Could you check a few things on this model? Use its own coordinates, in mm. Face numbers are marked on the shaded views. A direction names the side the tool comes from. Round coordinates to 2 decimals unless told otherwise and drop trailing zeros. Loops run counter-clockwise (first coordinate to the right, second up) from the corner with the lowest first, then second, coordinate; pieces in that order, holes last. Notation, with made-up numbers: (23, 46) -> (79, 46) arc R20 ccw to (79, 61) -> close; hole circle Ø6 at (14.5, -32.5). An arc over 180 degrees is marked (long way). One line per item, written item: value.
from build123d import *

# Parameters (mm, degrees)
BOSS_EXTRUDE1_DEPTH = 300
SKETCH3_W           = 90
SKETCH3_H           = 90
BOSS_EXTRUDE2_DEPTH = 70


with BuildPart() as part:
    # Sketch2 → Boss-Extrude1 (new body)
    with BuildSketch(Plane(origin=(0, 0, 0), x_dir=(1, 0, 0), z_dir=(0, 1, 0))):
        Polygon((0, 0), (0, 75), (45, 75), (110.363656587, 121.756282785), (145.853333333, 72.142949451), (45, 0), align=None)
    boss_extrude1 = extrude(amount=BOSS_EXTRUDE1_DEPTH)

    # Mirror1: Boss-Extrude1 across plane
    add(boss_extrude1.mirror(Plane(origin=(0, 0, 0), x_dir=(0, 0, 1), z_dir=(1, 0, 0))))

    # Sketch3 → Boss-Extrude2 (add)
    with BuildSketch(Plane.XY):
        with Locations((0, 255)):
            Rectangle(SKETCH3_W, SKETCH3_H)
    extrude(amount=BOSS_EXTRUDE2_DEPTH)


solid = part.part
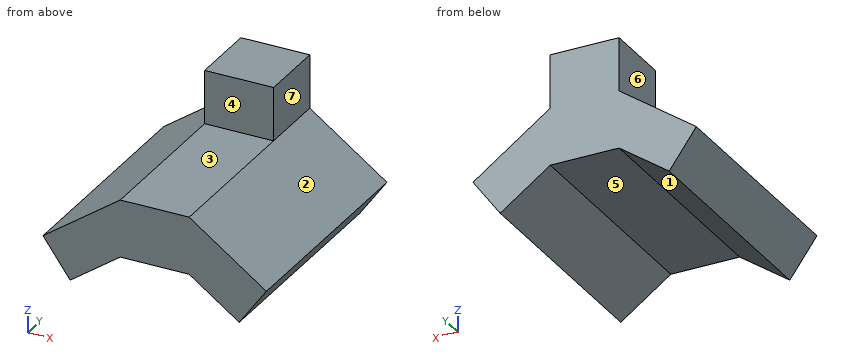
(1) If we section it at C-C, the plane z = -91: Please give me the cut outline in (x, y), then the cut area to 3 significant figures.
Recorded:
outline: (-132.36, 0) -> (-67.37, 0) -> (-67.37, 300) -> (-132.36, 300) -> close; (67.37, 0) -> (132.36, 0) -> (132.36, 300) -> (67.37, 300) -> close
area: 39,000 mm²
(2) If we section it at A-A, the plane y = 89: Please give me the cut outline in (x, z).
Recorded:
outline: (-145.85, -72.14) -> (-110.36, -121.76) -> (-45, -75) -> (45, -75) -> (110.36, -121.76) -> (145.85, -72.14) -> (45, 0) -> (-45, 0) -> close
(3) If we section it at D-D, the plane z = 55: Please give me the cut outline in (x, y), then the cut area to 3 significant figures.
Recorded:
outline: (-45, 210) -> (45, 210) -> (45, 300) -> (-45, 300) -> close
area: 8,100 mm²
(4) I'm going to push flat-ended pins straight in: pin 1 Ø1.5 at (y, z) = (61.5, -5) entering from -X; pin 2 Ø12 at (y, z) = (170.5, -93.5) entering from -X; pin 3 Ø5 at (y, z) = (157.5, -71) entering from +X. Where does each tip first touch, or does it pass through?
Recorded:
pin 1: x = -53.04
pin 2: x = -134.87
pin 3: x = 145.85
(5) Thinking about a two-plate mould opening in X: for the marked faces 1, 2 and 3, which applies, released by +X, released by -X, zero draft, split by the parting line, or undercut?
Recorded:
face 1: undercut
face 2: released by +X
face 3: zero draft
(6) For the marked faces 4, 5, 6 and 7, which set-ups out of +Z, -Z, +X, -X, +Y, -Y let a thin tool reach every point of the face, with its end or its side?
Recorded:
face 4: +Z, +X, -X, -Y
face 5: -Z, +Y, -Y
face 6: +Z, -X, +Y, -Y
face 7: +Z, +X, +Y, -Y
(7) If I drill on L1, parallel to Z at x = 22, y = 71.5; L2, parallel to X at y = 36, z = -111; L3, parallel to X at y = 229, z = 10, over which ranges is the centre line in solid material (lowest first)?
Recorded:
L1: -75 to 0
L2: -118.06 to -95.33, 95.33 to 118.06
L3: -45 to 45
(8) If we section it at B-B, the plane x = 36: Please give me the cut outline in (y, z).
Recorded:
outline: (0, -75) -> (300, -75) -> (300, 70) -> (210, 70) -> (210, 0) -> (0, 0) -> close
